Job drawing, mm, ordinate dimensions from the low corner. One solid piece. A direction names the side the tool comes from. Round coordinates to 2 decimals unless told otherwise and drop trailing zeros. Loops run counter-clockwise (first coordinate to the right, second up) from the corner with the lowest first, then second, coordinate; pieces in that order, holes last. Notation, with made-up numbers: M -1.5,37 L 39.5,37 A26 ccw 39.5,67 Z; hole C 87,88 d2. An arc over 180 degrees is marked long. Use a Markdown table: item, result. Add a question column.
(1) Wall check: L1, parallel to X at y = 26, z = 0.3; L2, parallel to X at y = 11.5, z = 0.1; L3, parallel to Y at x = 24.25, z = 2.7 (3 decimals). Give the ranges that are in metal, low to high.
(2) Band-saw the part on A-A, the plane z = 0.9. Write the cut outline in (x, y) (3 decimals).
(3) Band-saw the part on B-B, the plane y = 35. Write the cut outline in (x, z).
(4) Flat gauge pins, fed straight in: P1, Ø0.9, axis at x = 1, z = 2.5, coming from the -Y side; P2, Ø0.9, axis at x = 23.5, z = 1.5, coming from the +Y side (3 decimals); P3, Ø1.5, axis at x = 4.5, z = 1, coming from the -Y side. Where does each tip first touch, or does it go through?
(5) Which spindle directions (+Z, -Z, +X, -X, +Y, -Y) get a long thin tool onto all of the face, cutting with end or side? Do the marked faces 1, 2 and 3. Say none if no direction does.
(6) Band-saw the part on C-C, the plane x = 23. Write the cut outline in (y, z) (3 decimals).
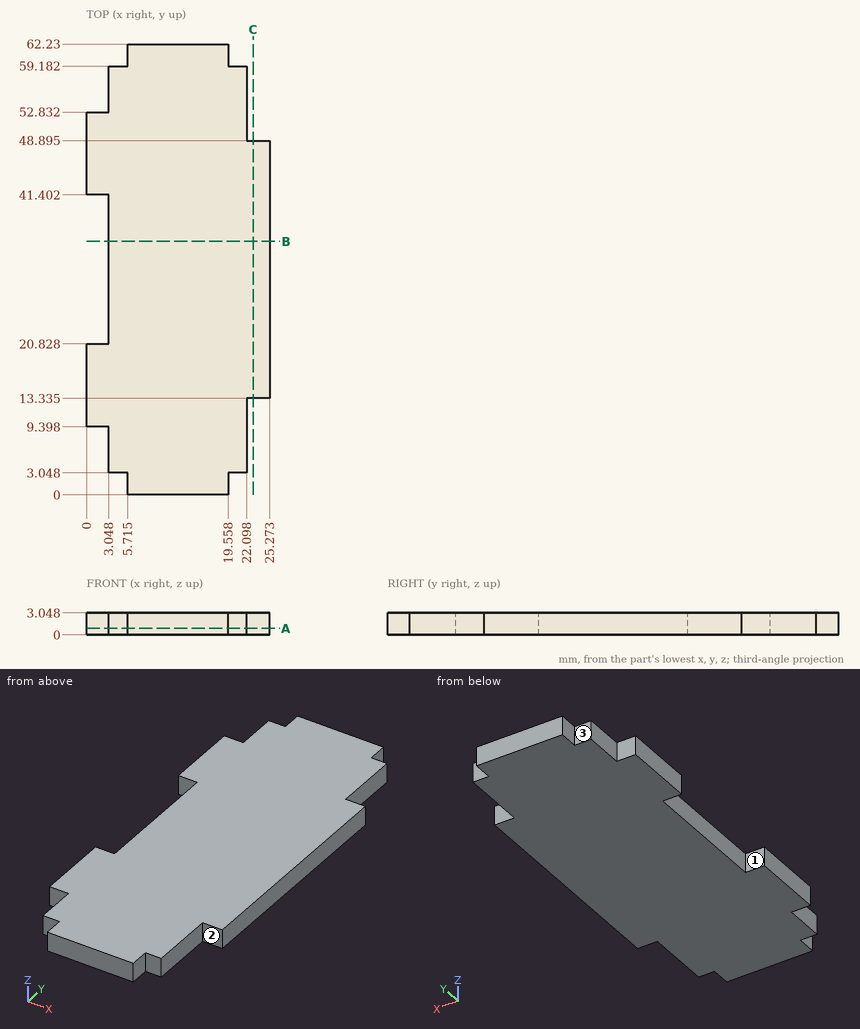
Return value:
| question | item | result |
|---|---|---|
| 1 | L1 | 3.05 to 25.27 |
| 1 | L2 | 0 to 22.1 |
| 1 | L3 | 13.335 to 48.895 |
| 2 | outline | M 0,9.398 L 3.048,9.398 L 3.048,3.048 L 5.715,3.048 L 5.715,0 L 19.558,0 L 19.558,3.048 L 22.098,3.048 L 22.098,13.335 L 25.273,13.335 L 25.273,48.895 L 22.098,48.895 L 22.098,59.182 L 19.558,59.182 L 19.558,62.23 L 5.715,62.23 L 5.715,59.182 L 3.048,59.182 L 3.048,52.832 L 0,52.832 L 0,41.402 L 3.048,41.402 L 3.048,20.828 L 0,20.828 Z |
| 3 | outline | M 3.05,0 L 25.27,0 L 25.27,3.05 L 3.05,3.05 Z |
| 4 | P1 | y = 9.4 |
| 4 | P2 | y = 48.895 |
| 4 | P3 | y = 3.05 |
| 5 | face 1 | +Z, -Z, -X |
| 5 | face 2 | +Z, -Z, +X, -Y |
| 5 | face 3 | +Z, -Z, -X, +Y |
| 6 | outline | M 13.335,0 L 48.895,0 L 48.895,3.048 L 13.335,3.048 Z |
